from build123d import *

# Parameters (mm, degrees)
BOSS_EXTRUDE1_DEPTH          = 53.975
F_10_0_1935_DIAMETER_HOLE1_D = 4.9149
CUT_EXTRUDE2_DEPTH           = 90.858670283
CUT_EXTRUDE3_START           = -3.175
SKETCH4_4_R                  = 2.45745
CUT_EXTRUDE3_DEPTH           = 3.175
CUT_EXTRUDE5_DEPTH           = 88.988181024
EXTRUDE_THIN1_DEPTH          = 50.8


with BuildPart() as part:
    # Sketch1 → Boss-Extrude1 (new body)
    with BuildSketch(Plane.XY):
        Polygon((0, 0), (50.8, 0), (50.8, 25.4), (25.4, 25.4), (25.4, 50.8), (0, 50.8), align=None)
    extrude(amount=BOSS_EXTRUDE1_DEPTH)

    # #10 (0.1935) Diameter Hole1 (through all)
    with Locations(Plane(origin=(12.319, 12.319, 53.975), x_dir=(1, 0, 0), z_dir=(0, 0, 1))):
        with Locations((0, 0)):
            Hole(F_10_0_1935_DIAMETER_HOLE1_D / 2)

    # Sketch4 → Cut-Extrude2 (cut, through all)
    with BuildSketch(Plane.XY.offset(53.975)):
        with BuildLine():
            ThreePointArc((12.7, 0), (3.719743879, 3.719743879), (0, 12.7))
            Line((0, 12.7), (0, 0))
            Line((0, 0), (12.7, 0))
        make_face()
    extrude(amount=-CUT_EXTRUDE2_DEPTH, mode=Mode.SUBTRACT)

    # Sketch4<4> → Cut-Extrude3 (cut)
    with BuildSketch(Plane.XY.offset(53.975).offset(CUT_EXTRUDE3_START)):
        with BuildLine():
            Line((25.4, 50.8), (7.571764462, 50.8))
            ThreePointArc((7.571764462, 50.8), (7.721601354, 49.175886193), (8.410645771, 47.697571429))
            ThreePointArc((8.410645771, 47.697571429), (9.549506799, 44.069), (8.410645771, 40.440428571))
            ThreePointArc((8.410645771, 40.440428571), (7.5565, 37.719), (8.410645771, 34.997571429))
            ThreePointArc((8.410645771, 34.997571429), (9.549506799, 31.369), (8.410645771, 27.740428571))
            ThreePointArc((8.410645771, 27.740428571), (7.5565, 25.019), (8.410645771, 22.297571429))
            ThreePointArc((8.410645771, 22.297571429), (9.549506799, 18.669), (8.410645771, 15.040428571))
            ThreePointArc((8.410645771, 15.040428571), (8.951403955, 8.951403955), (15.040428571, 8.410645771))
            ThreePointArc((15.040428571, 8.410645771), (16.767452272, 9.258105336), (18.669, 9.549506799))
            ThreePointArc((18.669, 9.549506799), (20.570547728, 9.258105336), (22.297571429, 8.410645771))
            ThreePointArc((22.297571429, 8.410645771), (25.019, 7.5565), (27.740428571, 8.410645771))
            ThreePointArc((27.740428571, 8.410645771), (29.467452272, 9.258105336), (31.369, 9.549506799))
            ThreePointArc((31.369, 9.549506799), (33.270547728, 9.258105336), (34.997571429, 8.410645771))
            ThreePointArc((34.997571429, 8.410645771), (37.719, 7.5565), (40.440428571, 8.410645771))
            ThreePointArc((40.440428571, 8.410645771), (42.167452272, 9.258105336), (44.069, 9.549506799))
            ThreePointArc((44.069, 9.549506799), (45.970547728, 9.258105336), (47.697571429, 8.410645771))
            ThreePointArc((47.697571429, 8.410645771), (49.175886193, 7.721601354), (50.8, 7.571764462))
            Line((50.8, 7.571764462), (50.8, 25.4))
            Line((50.8, 25.4), (25.4, 25.4))
            Line((25.4, 25.4), (25.4, 50.8))
        make_face()
        with Locations((12.319, 12.319)):
            Circle(SKETCH4_4_R, mode=Mode.SUBTRACT)
    extrude(amount=CUT_EXTRUDE3_DEPTH, mode=Mode.SUBTRACT)

    # Sketch7 → Cut-Extrude5 (cut, through all)
    with BuildSketch(Plane.XY.offset(50.8)):
        with BuildLine():
            Line((25.4, 50.8), (12.954, 50.8))
            ThreePointArc((12.954, 50.8), (17.900023052, 39.035105247), (25.4, 28.709107069))
            Line((25.4, 28.709107069), (25.4, 50.8))
        make_face()
        with BuildLine():
            Line((50.8, 25.4), (28.709107069, 25.4))
            ThreePointArc((28.709107069, 25.4), (39.035105247, 17.900023052), (50.8, 12.954))
            Line((50.8, 12.954), (50.8, 25.4))
        make_face()
    extrude(amount=-CUT_EXTRUDE5_DEPTH, mode=Mode.SUBTRACT)

    # Sketch8 → Extrude-Thin1 (add)
    with BuildSketch(Plane.XY.offset(50.8)):
        with BuildLine():
            ThreePointArc((25.4, 28.709107069), (27.019699139, 27.019699139), (28.709107069, 25.4))
            Line((28.709107069, 25.4), (26.990285921, 23.529905387))
            ThreePointArc((26.990285921, 23.529905387), (25.223647915, 25.223647915), (23.529905387, 26.990285921))
            Line((23.529905387, 26.990285921), (25.4, 28.709107069))
        make_face()
    extrude(amount=-EXTRUDE_THIN1_DEPTH)


solid = part.part
The listing builds one solid part. Answer for the finished solid, in the listing's coordinates (mm). A direction names the side the tool comes from. Round coordinates to 2 decimals unless told otherwise and drop trailing zeros. Order: outer loops, then holes, each group sorted by start corner. A loop starts at its lowest first (then second) coordinate and runs counter-clockwise, first axis right, second up. Notation, with made-up numbers: (27, 63) -> (40, 63) arc R10 cw to (40, 69) -> close; hole circle Ø6 at (-35.5, -38.5). An arc over 180 degrees is marked (long way). One line per item, written item: value.
Item 1: Find section D-D, the plane x = 4. Give the vertices of the cut face in (y, z) (3 decimals), then the cut area to 3 significant figures.
Taken from the geometry:
outline: (3.448, 0) -> (50.8, 0) -> (50.8, 53.975) -> (3.448, 53.975) -> close
area: 2,560 mm2
Item 2: Straight lines are drawn through the part: L1, parallel to X at y = 12.5, z = 18; L2, parallel to Z at x = 29, y = 18; L3, parallel to Y at x = 12, z = 37.5. For each, find the intervals that lie inside material, in ascending order.
Taken from the geometry:
L1: x = 0 to 9.87, 14.77 to 50.8
L2: z = 0 to 50.8
L3: y = 0.02 to 9.88, 14.76 to 50.8
Item 3: Find section A-A, the plane z = 32.5. Give the vertices of the cut face in (x, y) (1 decimal), then the cut area to 3 significant figures.
Taken from the geometry:
outline: (0, 12.7) arc R12.7 ccw to (12.7, 0) -> (50.8, 0) -> (50.8, 13) arc R55.6 cw to (13, 50.8) -> (0, 50.8) -> close; hole circle Ø4.9 at (12.3, 12.3)
area: 1,560 mm2
Item 4: For faces 1 (the cylindrical face through (8.886, 9.018, 52.365)), 2 (the cylindrical face through (37.678, 7.557, 52.365)), 3 (the cylindrical face through (7.716, 49.198, 52.365)), determine the directions among +Z, -Z, +X, -X, +Y, -Y from which every point of the face is accessible in a straight line to the end or side of a thin tool.
Taken from the geometry:
face 1: +Z
face 2: +Z, +Y
face 3: +Z, +X
Item 5: Find section C-C, the plane x = 46. Give the vertices of the cut face in (y, z) (3 decimals).
Taken from the geometry:
outline: (0, 0) -> (14.59, 0) -> (14.59, 50.8) -> (9.249, 50.8) -> (9.249, 53.975) -> (0, 53.975) -> close
Item 6: Find section B-B, the plane y = 18. Give the vertices of the cut face in (x, z) (3 decimals).
Taken from the geometry:
outline: (0, 0) -> (38.858, 0) -> (38.858, 50.8) -> (9.514, 50.8) -> (9.514, 53.975) -> (0, 53.975) -> close
Item 7: For a pull along X with two mould halves and no side action, classify faces 4 (the cylindrical face through (10.05, 11.38, 25.04)), 5 (the cylindrical face through (7.557, 37.76, 52.365)), 6 (the flat face through (20, 20, 0)) as released by +X, released by -X, zero draft, split by the parting line, or undercut.
Taken from the geometry:
face 4: undercut
face 5: released by +X
face 6: zero draft
Item 8: Given P1, Ø5.5, axis at x = 12.319, y = 12.319, coming from the +Z side; P2, Ø4, axis at y = 18.5, z = 47, coming from the +X side, each flat-ended and moving along its own axis, determine where each tip first touches the part or whether it passes through.
Taken from the geometry:
P1: stops at z = 50.8
P2: stops at x = 41.68
